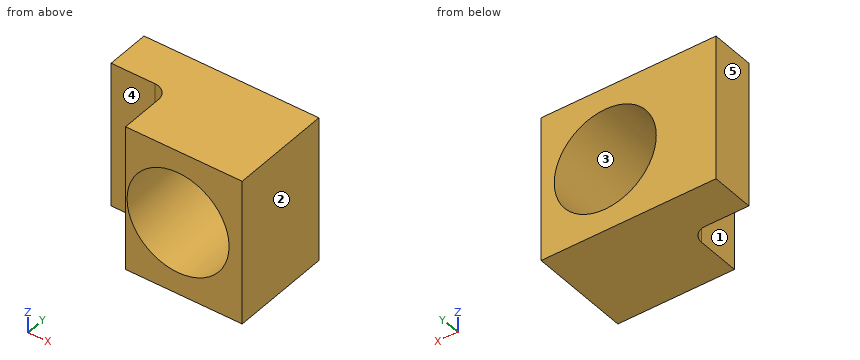
```python
from build123d import *

# Parameters (mm, degrees)
F1_DEPTH = 5
F2_R     = 1.75
F3_DEPTH = 25


with BuildPart() as f1:
    # F0 (on Top) → F1 (new body)
    with BuildSketch(Plane.XY):
        with BuildLine():
            Line((-4, 0), (0, 0))
            Line((0, 0), (0, 3.5))
            Line((0, 3.5), (-6, 3.5))
            Line((-6, 3.5), (-6, 2))
            Line((-6, 2), (-4.5, 2))
            ThreePointArc((-4.5, 2), (-4.146447, 1.853553), (-4, 1.5))
            Line((-4, 1.5), (-4, 0))
        make_face()
    extrude(amount=F1_DEPTH)

    # F2 (on face) → F3 (cut)
    with BuildSketch(Plane(origin=(0, 3.5, 0), x_dir=(-1, 0, 0), z_dir=(0, 1, 0))):
        with Locations((2.2, 2.5)):
            Circle(F2_R)
    extrude(amount=-F3_DEPTH, mode=Mode.SUBTRACT)


solid = f1.part
```
Build history of the part. All positions in model axes, mm. Face numbers are marked on the shaded views. A direction names the side the tool comes from. Give positions to 0.01 mm unless a question says otherwise; leave off trailing zeros. Order: outer loops, then holes, each group sorted by start corner. A loop starts at its lowest first (then second) coordinate and runs counter-clockwise, first axis right, second up. Notation, with made-up numbers: M -21,52 L -11,52 A29 ccw -11,83 Z; hole C 13.25,24.5 d1. An arc over 180 degrees is marked long. Write item = value, one per line. Start each with the question number.
(1) Two-plate mould, pull along X, no slides. Class the marked faces 1, 2 and 3: released by +X, released by -X, zero draft, split by the parting line, or undercut.
(2) Slice it at B-B on x = -2.2. Write the cut outline in (y, z), plus the area to 3 significant figures.
(3) Probe L1, parallel to Z at x = -2.2, y = 0.7; L2, parallel to Z at x = -2.8, y = 1.1; L3, parallel to X at y = 2.6, z = 1.6. List the from-to ranges inside material, lowest first. Write a range as [from, to].
(4) Slice it at C-C on y = 1.2. Write the cut outline in (x, z), plus the area to 3 significant figures.
(5) Slice it at D-D on y = 3.05. Write the cut outline in (x, z).
(6) Pin check, flat tips, straight feed: pin 1 Ø3 at (x, z) = (-2.2, 2.5) entering from -Y; pin 2 Ø0.8 at (y, z) = (1, 2.5) entering from -X. Stop position of each tip, or through.
(7) Slice it at A-A on z = 2.5. Write the cut outline in (x, y).
(8) Which spindle directions (+Z, -Z, +X, -X, +Y, -Y) get a long thin tool onto all of the face, cutting with end or side? Do the marked faces 4 and 5. Say none if no direction does.
Responses:
q1.face_1 = released by -X
q1.face_2 = released by +X
q1.face_3 = undercut
q2.outline = M 0,0 L 3.5,0 L 3.5,0.75 L 0,0.75 Z; M 0,4.25 L 3.5,4.25 L 3.5,5 L 0,5 Z
q2.area = 5.25 mm2
q3.L1 = [0, 0.75], [4.25, 5]
q3.L2 = [0, 0.86], [4.14, 5]
q3.L3 = [-6, -3.7], [-0.7, 0]
q4.outline = M -4,0 L 0,0 L 0,5 L -4,5 Z; hole C -2.2,2.5 d3.5
q4.area = 10.4 mm2
q5.outline = M -6,0 L 0,0 L 0,5 L -6,5 Z; hole C -2.2,2.5 d3.5
q6.pin_1 = through
q6.pin_2 = -4
q7.outline = M -6,2 L -4.5,2 A0.5 cw -4,1.5 L -4,0 L -3.95,0 L -3.95,3.5 L -6,3.5 Z; M -0.45,0 L 0,0 L 0,3.5 L -0.45,3.5 Z
q8.face_4 = +Z, -Z, -X, -Y
q8.face_5 = +Z, -Z, -X, +Y, -Y
